from build123d import *

# Parameters (mm, degrees)
SKETCH1_R           = 49
SKETCH1_R_2         = 2.5
SKETCH1_R_3         = 5
BOSS_EXTRUDE1_DEPTH = 76


with BuildPart() as part:
    # Sketch1 → Boss-Extrude1 (new body)
    with BuildSketch(Plane.XY):
        Circle(SKETCH1_R)
        with Locations((-30, 29.915097225)):
            Circle(SKETCH1_R_2, mode=Mode.SUBTRACT)
        with Locations((30, 29.915097225)):
            Circle(SKETCH1_R_3, mode=Mode.SUBTRACT)
        with Locations((-29.89855214, -30.18007542)):
            Circle(SKETCH1_R_2, mode=Mode.SUBTRACT)
        with Locations((30.10144786, -30.08971898)):
            Circle(SKETCH1_R_3, mode=Mode.SUBTRACT)
        with BuildLine():
            ThreePointArc((-15.874507866, -0.084902775), (0, -42.084902775), (15.874507866, -0.084902775))
            ThreePointArc((15.874507866, -0.084902775), (0, 41.915097225), (-15.874507866, -0.084902775))
        make_face(mode=Mode.SUBTRACT)
    extrude(amount=BOSS_EXTRUDE1_DEPTH)


solid = part.part
Geometry: final body of the model. Coordinates: model frame, mm. Give positions to 0.01 mm unless a question says otherwise; leave off trailing zeros. Order: outer loops, then holes, each group sorted by start corner. A loop starts at its lowest first (then second) coordinate and runs counter-clockwise, first axis right, second up. Notation, with made-up numbers: (5.25, -19.75) -> (11.25, -19.75) arc R31 ccw to (11.25, 17.25) -> close; hole circle Ø2 at (-24.75, -19). An arc over 180 degrees is marked (long way). Answer as a JSON object with one key per item and string values.
Q1. Section C-C (x = 30). Output: boundary loops of the cut face in (y, z).
Entries:
{"outline": "(-38.74, 0) -> (-35.09, 0) -> (-35.09, 76) -> (-38.74, 76) -> close; (-25.09, 0) -> (24.92, 0) -> (24.92, 76) -> (-25.09, 76) -> close; (34.92, 0) -> (38.74, 0) -> (38.74, 76) -> (34.92, 76) -> close"}
Q2. Section D-D (z = 55). Output: boundary loops of the cut face in (x, y).
Entries:
{"outline": "circle Ø98 at (0, 0); hole circle Ø5 at (-30, 29.92); hole circle Ø5 at (-29.9, -30.18); hole (-15.87, -0.08) arc R24 ccw (long way) to (15.87, -0.08) arc R24 ccw (long way) to start; hole circle Ø10 at (30, 29.92); hole circle Ø10 at (30.1, -30.09)"}
Q3. Material intervals for probe 1 along Y at (x, z) = (17, 46.5); probe 2 along X at (y, z) = (-29.5, 72); probe 3 along Y at (x, z) = (30, 25), sorted ascending.
Entries:
{"probe 1": "y = -45.96 to -35.03, -1.14 to 0.97, 34.86 to 45.96", "probe 2": "x = -39.12 to -32.3, -27.49 to -21.11, 21.11 to 25.14, 35.07 to 39.12", "probe 3": "y = -38.74 to -35.09, -25.09 to 24.92, 34.92 to 38.74"}
Q4. Draft query along X for faces 1 (the cylindrical face through (26.34, 41.32, 37.47)), 2 (the cylindrical face through (-30.542, 27.475, 37.468)), 3 (the cylindrical face through (0.8, 41.9, 37.5)), 4 (the flat face through (21, 1, 76)). Return one class per face: released by +X, released by -X, zero draft, split by the parting line, or undercut.
Entries:
{"face 1": "split by the parting line", "face 2": "undercut", "face 3": "undercut", "face 4": "zero draft"}
Q5. First-contact query: pin 1 (5 mm diameter, centred on x = 12.5, z = 34.5, fed in from +Y); pin 2 (3 mm diameter, centred on y = 22.5, z = 48.5, fed in from +X); pin 3 (1.5 mm diameter, centred on x = 23, z = 56.5, fed in from +Y). Flat tips, straight axial feed; report the tip coordinate or a pass-through.
Entries:
{"pin 1": "stops at y = 47.97", "pin 2": "stops at x = 44.27", "pin 3": "stops at y = 43.66"}
Q6. Section A-A (x = 0). Output: boundary loops of the cut face in (y, z), plus the area to 3 significant figures.
Entries:
{"outline": "(-49, 0) -> (-42.08, 0) -> (-42.08, 76) -> (-49, 76) -> close; (41.92, 0) -> (49, 0) -> (49, 76) -> (41.92, 76) -> close", "area": "1,060 mm^2"}
Q7. Section B-B (y = 19.5). Output: boundary loops of the cut face in (x, z).
Entries:
{"outline": "(-44.95, 0) -> (-23.95, 0) -> (-23.95, 76) -> (-44.95, 76) -> close; (23.95, 0) -> (44.95, 0) -> (44.95, 76) -> (23.95, 76) -> close"}
